Could you check a few things on this model? Use its own coordinates, in mm. A direction names the side the tool comes from. Round coordinates to 2 decimals unless told otherwise and drop trailing zeros. Loops run counter-clockwise (first coordinate to the right, second up) from the corner with the lowest first, then second, coordinate; pieces in that order, holes last. Notation, with made-up numbers: M -36.5,-2 L -18.5,-2 A29 ccw -18.5,32 Z; hole C 15,61 d3. An arc over 180 degrees is marked long. One line per item, written item: value. Start each with the question number.
Q1. Which directions (+Z, -Z, +X, -X, +Y, -Y) give clear straight access to the entire face, cutting with the end or side of a thin tool? Please do faces 1 (the face through (-23.146, 8.676, 9.36)), 2 (the face through (0, 15, -19.5)).
Q2. Thinking about a two-plate mould opening in Y: for faces 3 (the face through (19.962, 20.004, 9.36)), 4 (the face through (25, 15, 3)), 5 (the face through (5, 0, 13)), which applies, released by +Y, released by -Y, zero draft, split by the parting line, or undercut?
Q3. Imagine slicing it at A-A (y = 17.5). Please give me the cut outline in (x, z).
Q4. Please list where these lines run through material, in increasing order: line 1 along X through (y, z) = (8, 6.75); line 2 along X through (y, z) = (8, 14); line 3 along X through (y, z) = (22, 9.5).
Q5. I'm going to push a flat-ended pin straight in: pin 1 Ø5 at (x, y) = (21, 22) entering from +Z. Where does the tip first touch, or does it pass through?
Q6. Imagine slicing it at C-C (x = -6.5). Please give me the cut outline in (y, z), then the cut area to 3 significant figures.
Q7. Imagine slicing it at B-B (z = 4.5). Please give me the cut outline in (x, y).
Q8. Imagine slicing it at D-D (z = -13). Please give me the cut outline in (x, y), then the cut area to 3 significant figures.
from build123d import *

# Parameters (mm, degrees)
SKETCH_1_W             = 50
SKETCH_1_H             = 39
EXTRUDE_1_DEPTH        = 30
SKETCH_2_R             = 15
CUT_EXTRUDE_1_DEPTH    = 30
CHAMFER_1_SIZE         = 5
HOLE_WIZARD_M4_1_D     = 4.5
HOLE_WIZARD_M4_1_DEPTH = 20
HOLE_WIZARD_M4_1_TIP   = 1.351936393


with BuildPart() as part:
    # 스케치1 → 보스-돌출1 (new body)
    with BuildSketch(Plane(origin=(0, 0, 0), x_dir=(1, 0, 0), z_dir=(0, 1, 0))):
        Rectangle(SKETCH_1_W, SKETCH_1_H)
    extrude(amount=EXTRUDE_1_DEPTH)

    # 스케치2 → 컷-돌출1 (cut)
    with BuildSketch(Plane(origin=(0, 30, 0), x_dir=(1, 0, 0), z_dir=(0, 1, 0))):
        with Locations(Location((0, 1.5, 0), (0, 0, 270))):
            Circle(SKETCH_2_R)
    extrude(amount=-CUT_EXTRUDE_1_DEPTH, mode=Mode.SUBTRACT)

    # 모따기1
    chamfer_1_edges = [part.edges().sort_by_distance(p)[0] for p in [
        (-25, 15, -19.5),
        (25, 15, -19.5),
    ]]
    chamfer(chamfer_1_edges, length=CHAMFER_1_SIZE)

    # M4 여유 구멍1
    with Locations(Plane.XY.offset(19.5)):
        with Locations((-21, 22), (21, 22), (21, 8), (-21, 8)):
            Hole(HOLE_WIZARD_M4_1_D / 2, depth=HOLE_WIZARD_M4_1_DEPTH)
            with Locations((0, 0, -(HOLE_WIZARD_M4_1_DEPTH + HOLE_WIZARD_M4_1_TIP / 2))):  # 118° drill point
                Cone(0, HOLE_WIZARD_M4_1_D / 2, HOLE_WIZARD_M4_1_TIP, mode=Mode.SUBTRACT)


solid = part.part
Report:
1. face 1: +Z
1. face 2: -Z, +X, -X, +Y, -Y
2. face 3: undercut
2. face 4: zero draft
2. face 5: released by -Y
3. outline: M -25,-14.5 L -20,-19.5 L 20,-19.5 L 25,-14.5 L 25,19.5 L -25,19.5 Z; hole C 0,-1.5 d30
4. line 1: x = -25 to -23.25, -18.75 to -12.53, 12.53 to 18.75, 23.25 to 25
4. line 2: x = -25 to -23.25, -18.75 to 18.75, 23.25 to 25
4. line 3: x = -25 to -23.25, -18.75 to -10.2, 10.2 to 18.75, 23.25 to 25
5. pin 1: stops at z = 19.5
6. outline: M 0,-19.5 L 30,-19.5 L 30,-15.02 L 0,-15.02 Z; M 0,12.02 L 30,12.02 L 30,19.5 L 0,19.5 Z
6. area: 359 mm²
7. outline: M -25,0 L -13.75,0 L -13.75,30 L -25,30 Z; M 13.75,0 L 25,0 L 25,30 L 13.75,30 Z; hole C -21,8 d4.5; hole C -21,22 d4.5; hole C 21,8 d4.5; hole C 21,22 d4.5
8. outline: M -25,0 L -9.63,0 L -9.63,30 L -25,30 Z; M 9.63,0 L 25,0 L 25,30 L 9.63,30 Z
8. area: 922 mm²
